Verification items for the finished model (mm, model axes). A direction names the side the tool comes from. Give positions to 0.01 mm unless a question says otherwise; leave off trailing zeros. Write each loop counter-clockwise with the first axis right and the second up, starting at its lowest first coordinate (ties: lowest second). Pieces come first, ordered by that corner, then holes. Notation, with made-up numbers: (59, -3.5) - (90, -3.5) arc R19 ccw to (90, 18.5) - close; hole circle Ø4 at (37.25, -4.5). An arc over 180 degrees is marked (long way). Answer as a JSON object with one key per item and string values. Group by question number.
Item 1: Sectioned sample at B-B, the plane z = 25.4. Record the boundary of the cut face in (x, y), and give its area (3 significant figures).
Item 2: Go/stop test with flat-tipped pins: pin 1 (5 mm diameter, centred on x = 23, z = -10.5, fed in from +Y); pin 2 (11.5 mm diameter, centred on x = 22, z = 12.7, fed in from -Y); pin 3 (15.5 mm diameter, centred on x = -5, z = 49, fed in from -Y). Record where each tip stops, or that it passes through.
Item 3: Tool access check on faces 1 (the face through (2, 4, -23)), 2 (the face through (-29.077, 7.395, -28.226)), 3 (the face through (0, -36, 65.5)). Record the directions out of +Z, -Z, +X, -X, +Y, -Y that give a thin tool (end or side, any length) a straight path to the whole face; none if there is none.
Item 4: Scan lines: line 1 along Z through (x, y) = (-24.5, -13); line 2 along X through (y, z) = (9, -30); line 3 along X through (y, z) = (10, -12). Record each from-to range of solid material in increasing order. Write a range as [from, to].
Item 5: Draft check along Z on faces 4 (the face through (24.1, 4, -10.5)), 5 (the face through (0, -70, 37)), 6 (the face through (-1, 2, -23)), 7 (the face through (0, 7, -35)). Enter one of: +Z half, -Z half, draft (parallel to the pull), parting line (faces both ways), or undercut.
Item 6: Sectioned sample at D-D, the plane y = 6.5. Count the separate pieces of the cut face and the enclosed holes in it, and give its area (3 significant figures).
Item 7: Sectioned sample at A-A, the plane z = 12.7. Record the boundary of the cut face in (x, y), and give its area (3 significant figures).
Item 8: Sectioned sample at C-C, the plane y = -49.5. Record the boundary of the cut face in (x, z), and give its area (3 significant figures).
```python
from build123d import *

# Parameters (mm, degrees)
SKETCH1_W           = 70
SKETCH1_H           = 70
SKETCH1_R           = 2.6
SKETCH1_R_2         = 10
SKETCH1_R_3         = 2
BOSS_EXTRUDE1_DEPTH = 15
SKETCH2_R           = 5
SKETCH2_R_2         = 2.6
CUT_EXTRUDE1_DEPTH  = 11
BOSS_EXTRUDE2_DEPTH = 70
FILLET1_R           = 5
FILLET2_R           = 1


with BuildPart() as part:
    # Sketch1 → Boss-Extrude1 (new body)
    with BuildSketch(Plane(origin=(0, 0, 0), x_dir=(1, 0, 0), z_dir=(0, 1, 0))):
        Rectangle(SKETCH1_W, SKETCH1_H)
        with Locations((0, 25.4)):
            Circle(SKETCH1_R, mode=Mode.SUBTRACT)
        with Locations((21.997045256, 12.7)):
            Circle(SKETCH1_R, mode=Mode.SUBTRACT)
        with Locations((21.997045256, -12.7)):
            Circle(SKETCH1_R, mode=Mode.SUBTRACT)
        with Locations((0, -25.4)):
            Circle(SKETCH1_R, mode=Mode.SUBTRACT)
        with Locations((-21.997045256, -12.7)):
            Circle(SKETCH1_R, mode=Mode.SUBTRACT)
        with Locations((-21.997045256, 12.7)):
            Circle(SKETCH1_R, mode=Mode.SUBTRACT)
        Circle(SKETCH1_R_2, mode=Mode.SUBTRACT)
        with Locations((-30, 30)):
            Circle(SKETCH1_R_3, mode=Mode.SUBTRACT)
        with Locations((30, 30)):
            Circle(SKETCH1_R_3, mode=Mode.SUBTRACT)
        with Locations((30, -30)):
            Circle(SKETCH1_R_3, mode=Mode.SUBTRACT)
        with Locations((-30, -30)):
            Circle(SKETCH1_R_3, mode=Mode.SUBTRACT)
    extrude(amount=BOSS_EXTRUDE1_DEPTH)

    # Sketch2 → Cut-Extrude1 (cut)
    with BuildSketch(Plane(origin=(0, 15, 0), x_dir=(1, 0, 0), z_dir=(0, 1, 0))):
        with Locations((-21.997045256, -12.7)):
            Circle(SKETCH2_R)
        with Locations((-21.997045256, -12.7)):
            Circle(SKETCH2_R_2, mode=Mode.SUBTRACT)
        with Locations((0, -25.4)):
            Circle(SKETCH2_R)
        with Locations((0, -25.4)):
            Circle(SKETCH2_R_2, mode=Mode.SUBTRACT)
        with Locations((21.997045256, -12.7)):
            Circle(SKETCH2_R)
        with Locations((21.997045256, -12.7)):
            Circle(SKETCH2_R_2, mode=Mode.SUBTRACT)
        with Locations((21.997045256, 12.7)):
            Circle(SKETCH2_R)
        with Locations((21.997045256, 12.7)):
            Circle(SKETCH2_R_2, mode=Mode.SUBTRACT)
        with Locations((0, 25.4)):
            Circle(SKETCH2_R)
        with Locations((0, 25.4)):
            Circle(SKETCH2_R_2, mode=Mode.SUBTRACT)
        with Locations((-21.997045256, 12.7)):
            Circle(SKETCH2_R)
        with Locations((-21.997045256, 12.7)):
            Circle(SKETCH2_R_2, mode=Mode.SUBTRACT)
    extrude(amount=-CUT_EXTRUDE1_DEPTH, mode=Mode.SUBTRACT)

    # Sketch3 → Boss-Extrude2 (add)
    with BuildSketch(Plane.ZY.offset(35)):
        with BuildLine():
            Line((35, 0), (35, -70))
            Line((35, -70), (40, -70))
            Line((40, -70), (40, -3))
            ThreePointArc((40, -3), (40.878679656, -0.878679656), (43, 0))
            Line((43, 0), (62.5, 0))
            ThreePointArc((62.5, 0), (64.621320344, -0.878679656), (65.5, -3))
            Line((65.5, -3), (65.5, -70))
            Line((65.5, -70), (70.5, -70))
            Line((70.5, -70), (70.5, 0))
            Line((70.5, 0), (70.5, 1))
            ThreePointArc((70.5, 1), (66.399494937, 10.899494937), (56.5, 15))
            Line((56.5, 15), (35, 15))
            Line((35, 15), (35, 0))
        make_face()
    extrude(amount=-BOSS_EXTRUDE2_DEPTH)

    # Fillet1
    fillet1_edges = [part.edges().sort_by_distance(p)[0] for p in [
        (-35, 7.5, -35),
        (35, 7.5, -35),
    ]]
    fillet(fillet1_edges, radius=FILLET1_R)

    # Fillet2
    fillet2_edges = [part.edges().sort_by_distance(p)[0] for p in [
        (0, -70, 70.5),
        (0, -70, 65.5),
        (0, -70, 40),
        (0, -70, 35),
    ]]
    fillet(fillet2_edges, radius=FILLET2_R)


solid = part.part
```
Geometry check:
{
 "1": {"outline": "(-35, 0) - (-2.6, 0) - (-2.6, 4) - (-5, 4) - (-5, 15) - (-35, 15) - close; (2.6, 0) - (35, 0) - (35, 15) - (5, 15) - (5, 4) - (2.6, 4) - close", "area": "919 mm^2"},
 "2": {"pin 1": "y = 4", "pin 2": "y = 0", "pin 3": "y = -0.56"},
 "3": {"face 1": "+Y", "face 2": "+Y, -Y", "face 3": "+X, -X, -Y"},
 "4": {"line 1": "[35, 40], [65.5, 70.5]", "line 2": "[-35, -32], [-28, -1.96], [1.96, 28], [32, 35]", "line 3": "[-35, -26.95], [-17.05, 17.05], [26.95, 35]"},
 "5": {"face 4": "undercut", "face 5": "draft", "face 6": "undercut", "face 7": "-Z half"},
 "6": {"separate pieces": "1", "enclosed holes": "11", "area": "6,460 mm^2"},
 "7": {"outline": "(-35, 0) - (-24.6, 0) - (-24.6, 4) - (-27, 4) - (-27, 15) - (-35, 15) - close; (-19.4, 0) - (19.4, 0) - (19.4, 4) - (17, 4) - (17, 15) - (-17, 15) - (-17, 4) - (-19.4, 4) - close; (24.6, 0) - (35, 0) - (35, 15) - (27, 15) - (27, 4) - (24.6, 4) - close", "area": "788 mm^2"},
 "8": {"outline": "(-35, 35) - (35, 35) - (35, 40) - (-35, 40) - close; (-35, 65.5) - (35, 65.5) - (35, 70.5) - (-35, 70.5) - close", "area": "700 mm^2"}
}
